The figure shows three views and two pictorial views of one solid part (mm, origin at its lowest corner). Answer the questions. A direction names the side the tool comes from. Coordinates: 2 decimals unless noted, no trailing zeros. Order: outer loops, then holes, each group sorted by start corner. A loop starts at its lowest first (then second) coordinate and runs counter-clockwise, first axis right, second up.
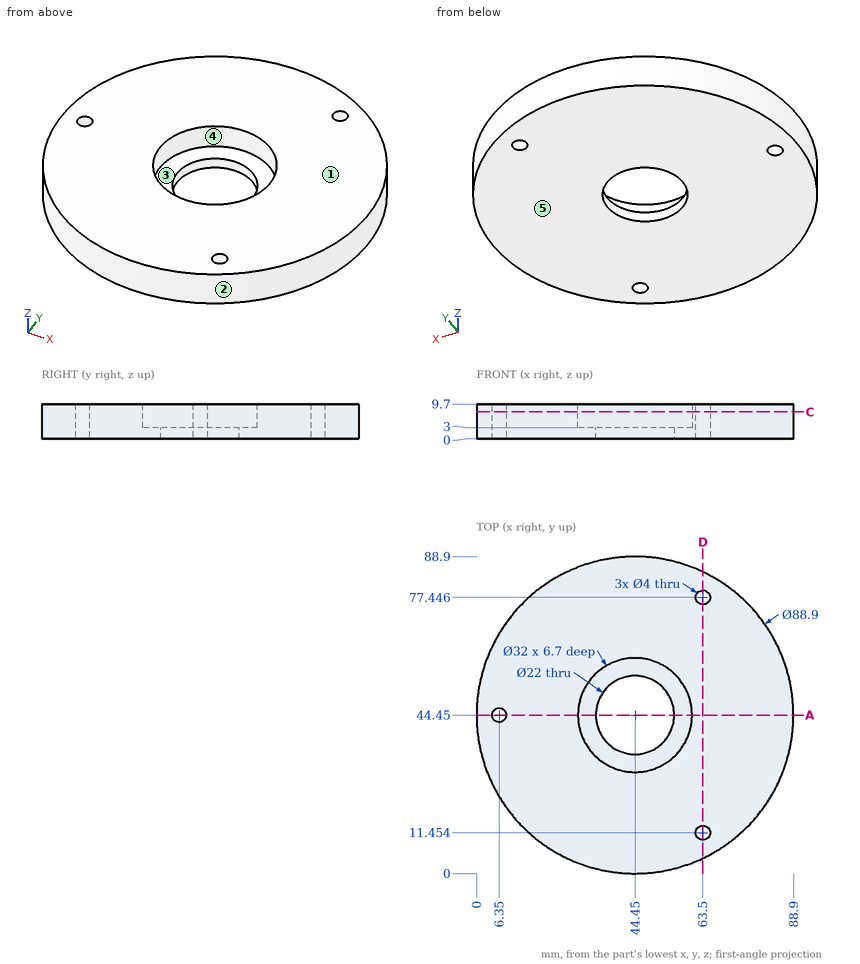
Q1. Each of these flat-tipped pins is pushed along its axis until it touches: P1, Ø1, axis at y = 41, z = 2.5, coming from the -X side; P2, Ø5, axis at x = 27, z = 7.5, coming from the -Y side; P3, Ø10, axis at x = 75.5, y = 51, coming from the -Z side; P4, Ø3, axis at x = 43, z = 8, coming from the -Y side. Where does it stop, or does it pass through?
Q2. The part is cut by section D-D, the plane x = 63.5. Determine the outline of the cut face in (y, z) (1 decimal).
Q3. Straight lines are drawn through the part: L1, parallel to Y at x = 44.45, z = 0.7; L2, parallel to Y at x = 63.5, z = 3 (1 decimal); L3, parallel to Y at x = 44.45, z = 7. For each, find the intervals that lie inside material, in ascending order.
Q4. The part is cut by section C-C, the plane z = 7.5. State how many separate pieces and enclosed holes the cut face has.
Q5. The part is cut by section A-A, the plane y = 44.45. Determine the outline of the cut face in (x, z), then the cut area to 3 significant figures.
Q6. Which of the six approach directions +Z, -Z, +X, -X, +Y, -Y give full straight-line access (tool end or side, diameter ignored) to the marked faces 4 and 5?
Q7. Determine the mould class of the marked faces 1, 2 and 3 for opening direction X: +X half, -X half, draft (parallel to the pull), parting line (faces both ways), or undercut.
Computed values:
1. P1: stops at x = 0.1
1. P2: stops at y = 2.59
1. P3: stops at z = 0
1. P4: stops at y = 0
2. outline: (4.3, 0) - (9.5, 0) - (9.5, 9.7) - (4.3, 9.7) - close; (13.5, 0) - (75.4, 0) - (75.4, 9.7) - (13.5, 9.7) - close; (79.4, 0) - (84.6, 0) - (84.6, 9.7) - (79.4, 9.7) - close
3. L1: y = 0 to 33.45, 55.45 to 88.9
3. L2: y = 4.3 to 9.5, 13.5 to 75.4, 79.4 to 84.6
3. L3: y = 0 to 28.45, 60.45 to 88.9
4. separate pieces: 1
4. enclosed holes: 4
5. outline: (0, 0) - (4.35, 0) - (4.35, 9.7) - (0, 9.7) - close; (8.35, 0) - (33.45, 0) - (33.45, 3) - (28.45, 3) - (28.45, 9.7) - (8.35, 9.7) - close; (55.45, 0) - (88.9, 0) - (88.9, 9.7) - (60.45, 9.7) - (60.45, 3) - (55.45, 3) - close
5. area: 543 mm2
6. face 4: +Z
6. face 5: -Z, +X, -X, +Y, -Y
7. face 1: draft
7. face 2: parting line
7. face 3: undercut
